The listing builds one solid part. Answer for the finished solid, in the listing's coordinates (mm). Face numbers are marked on the shaded views. A direction names the side the tool comes from. Coordinates: 2 decimals unless noted, no trailing zeros. Loops run counter-clockwise (first coordinate to the right, second up) from the corner with the lowest first, then second, coordinate; pieces in that order, holes last. Notation, with made-up numbers: M 40.5,-7.75 L 48.5,-7.75 A36 ccw 48.5,26.25 Z; hole C 72,33.5 d9. An arc over 180 degrees is marked long. Answer as a JSON object with one key per item and string values. Group by question number.
1. A cutting plane is placed at B-B on x = -0.5. Give the vertices of the cut face in (y, z).
2. Given pin 1 (6 mm diameter, centred on x = -3.5, y = 14, fed in from +Z); pin 2 (1.6 mm diameter, centred on x = 2.5, z = 9, fed in from -Y); pin 3 (1.5 mm diameter, centred on x = 1, z = 13, fed in from +Y); pin 4 (3.5 mm diameter, centred on y = -2, z = 10, fed in from +X), each flat-ended and moving along its own axis, determine where each tip first touches the part or whether it passes through.
3. A cutting plane is placed at D-D on x = 2.5. Give the vertices of the cut face in (y, z), and give its area (3 significant figures).
4. Straight lines are drawn through the part: L1, parallel to Z at x = 2.5, y = 6; L2, parallel to Y at x = 2.25, z = 8.5; L3, parallel to Y at x = 1.75, z = 7.5. For each, find the intervals that lie inside material, in ascending order.
5. For the marked faces 1 and 2, determine the directions among +Z, -Z, +X, -X, +Y, -Y from which every point of the face is accessible in a straight line to the end or side of a thin tool.
6. A cutting plane is placed at C-C on y = -1.75. Give the vertices of the cut face in (x, z), and give its area (3 significant figures).
7. A cutting plane is placed at A-A on z = 4. Give the vertices of the cut face in (x, y), and give its area (3 significant figures).
from build123d import *

# Parameters (mm, degrees)
F1_DEPTH = 15
F3_D     = 2.9
F3_DEPTH = 10
F3_TIP   = 0.8712478976
F4_SIZE2 = 3
F4_SIZE  = 1.5
F5_R     = 3


with BuildPart() as f1:
    # F0 (on Top) → F1 (new body)
    with BuildSketch(Plane.XY):
        Polygon((0, 0), (5.5, 0), (5.5, 18), (-6, 18), (-6, -10), (0, -10), align=None)
    extrude(amount=F1_DEPTH)

    # F3
    with Locations(Plane.YZ.offset(5.5)):
        with Locations((6, 7.5), (12, 7.5)):
            Hole(F3_D / 2, depth=F3_DEPTH)
            with Locations((0, 0, -(F3_DEPTH + F3_TIP / 2))):  # 118° drill point
                Cone(0, F3_D / 2, F3_TIP, mode=Mode.SUBTRACT)

    # F4
    f4_edges = [f1.edges().sort_by_distance(p)[0] for p in [
        (0, -10, 7.5),
    ]]
    f4_side = f1.faces().sort_by_distance((-3, -10, 7.5))[0]
    chamfer(f4_edges, length=F4_SIZE, length2=F4_SIZE2, reference=f4_side)

    # F5
    f5_edges = [f1.edges().sort_by_distance(p)[0] for p in [
        (-0.25, 18, 15),
        (-0.25, 18, 0),
        (-6, 18, 7.5),
        (-6, 4, 0),
        (-6, 4, 15),
        (-6, -10, 7.5),
    ]]
    fillet(f5_edges, radius=F5_R)


solid = f1.part
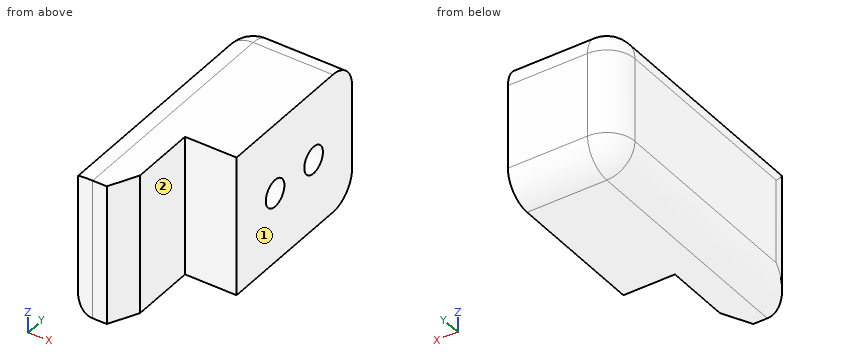
From the geometry:
{
 "1": {"outline": "M -8,0 L 15,0 A3 ccw 18,3 L 18,12 A3 ccw 15,15 L -8,15 Z; hole C 6,7.5 d2.9; hole C 12,7.5 d2.9"},
 "2": {"pin 1": "stops at z = 15", "pin 2": "stops at y = 0", "pin 3": "stops at y = 17.99", "pin 4": "stops at x = 0"},
 "3": {"outline": "M 0,0 L 15,0 A3 ccw 18,3 L 18,12 A3 ccw 15,15 L 0,15 Z; hole C 6,7.5 d2.9; hole C 12,7.5 d2.9", "area": "253 mm²"},
 "4": {"L1": "z = 0 to 6.05, 8.95 to 15", "L2": "y = 0 to 4.95, 7.05 to 10.95, 13.05 to 18", "L3": "y = 0 to 4.55, 7.45 to 10.55, 13.45 to 18"},
 "5": {"face 1": "+Z, -Z, +X, +Y, -Y", "face 2": "+Z, -Z, +X, -Y"},
 "6": {"outline": "M -6,3 A3 ccw -3,0 L 0,0 L 0,15 L -3,15 A3 ccw -6,12 Z", "area": "86.1 mm²"},
 "7": {"outline": "M -6,-7 A3 ccw -3,-10 L -1.5,-10 L 0,-7 L 0,0 L 5.5,0 L 5.5,18 L -3,18 A3 ccw -6,15 Z", "area": "261 mm²"}
}
